Model file for the job. Use its own axes, mm. Face numbers are marked on the shaded views. A direction names the side the tool comes from. Give positions to 0.01 mm unless a question says otherwise; leave off trailing zeros. Write each loop counter-clockwise with the first axis right and the second up, starting at its lowest first coordinate (ties: lowest second). Pieces come first, ordered by that corner, then holes. Notation, with made-up numbers: (71.5, 63) - (94.5, 63) arc R15 cw to (94.5, 90) - close; hole circle Ø4 at (41.5, 53). An arc over 180 degrees is marked (long way). Use a Markdown table: item, result. Add a question column.
```python
from build123d import *

# Parameters (mm, degrees)
ESBO_O1_R                = 1.5
RESSALTO_EXTRUS_O1_DEPTH = 50
ESBO_O2_R                = 2.5
ESBO_O2_W                = 6
ESBO_O2_H                = 10
CORTE_EXTRUS_O2_DEPTH    = 6


with BuildPart() as part:
    # Esboço1 → Ressalto-extrusão1 (new body)
    with BuildSketch(Plane.XY):
        with BuildLine():
            Line((0, 0), (-20, 0))
            ThreePointArc((-20, 0), (-22.324602514, 3.419903881), (-18.2892713, 4.32302148))
            ThreePointArc((-18.2892713, 4.32302148), (-17.800459182, 3.688284557), (-17.537523452, 2.9315197))
            ThreePointArc((-17.537523452, 2.9315197), (-16.656985327, 1.403588896), (-15, 0.8))
            Line((-15, 0.8), (0, 0.8))
            Line((0, 0.8), (0, 0))
        make_face()
        with Locations((-20, 2.5)):
            Circle(ESBO_O1_R, mode=Mode.SUBTRACT)
    extrude(amount=RESSALTO_EXTRUS_O1_DEPTH)

    # Esboço2 → Corte-extrusão2 (cut, through all)
    with BuildSketch(Plane.XZ):
        with Locations((-8, 43)):
            Circle(ESBO_O2_R)
        with Locations((-8, 7)):
            Circle(ESBO_O2_R)
        with Locations((-19.5, 5)):
            Rectangle(ESBO_O2_W, ESBO_O2_H)
        with Locations((-19.5, 25)):
            Rectangle(ESBO_O2_W, ESBO_O2_H)
        with Locations((-19.5, 45)):
            Rectangle(ESBO_O2_W, ESBO_O2_H)
    extrude(amount=-CORTE_EXTRUS_O2_DEPTH, mode=Mode.SUBTRACT)


solid = part.part
```
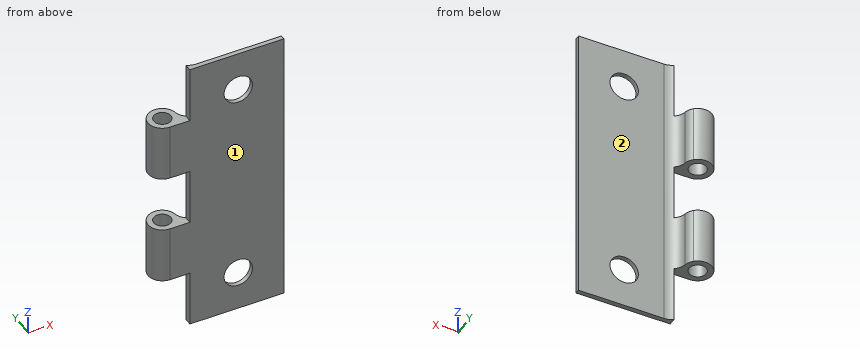
(1) Flat gauge pins, fed straight in: pin 1 (1.4 mm diameter, centred on y = 0.5, z = 25.5, fed in from -X); pin 2 (2.5 mm diameter, centred on x = -18.5, y = 3.5, fed in from -Z); pin 3 (2.5 mm diameter, centred on x = -20, y = 2.5, fed in from +Z); pin 4 (12 mm diameter, centred on x = -10, z = 23, fed in from +Y). Where does each tip first touch, or does it go through?
(2) Probe probe 1 along Z at (x, y) = (-8, 0.25); probe 2 along Z at (x, y) = (-7.25, 0.7); probe 3 along Z at (x, y) = (-21, 0.45). List the from-to ranges inside material, lowest first. Write a range as [from, to].
(3) Band-saw the part on D-D (z = 47). Write the cut outline in (x, y).
(4) Band-saw the part on B-B (x = -8). Write the cut outline in (y, z), then the cut area to 3 significant figures.
(5) Which spindle directions (+Z, -Z, +X, -X, +Y, -Y) get a long thin tool onto all of the face, cutting with end or side? Do the marked faces 1 and 2. Say none if no direction does.
(6) Band-saw the part on C-C (x = -17). Write the cut outline in (y, z), then the cut area to 3 significant figures.
(7) Band-saw the part on A-A (z = 5). Write the cut outline in (x, y).
Model answer:
| question | item | result |
|---|---|---|
| 1 | pin 1 | stops at x = -16.5 |
| 1 | pin 2 | stops at z = 10 |
| 1 | pin 3 | passes through |
| 1 | pin 4 | stops at y = 1 |
| 2 | probe 1 | z = [0, 4.5], [9.5, 40.5], [45.5, 50] |
| 2 | probe 2 | z = [0, 4.62], [9.38, 40.62], [45.38, 50] |
| 2 | probe 3 | z = [10, 20], [30, 40] |
| 3 | outline | (-16.5, 0) - (0, 0) - (0, 0.8) - (-15, 0.8) arc R2.58 cw to (-16.5, 1.28) - close |
| 4 | outline | (0, 0) - (0.8, 0) - (0.8, 4.5) - (0, 4.5) - close; (0, 9.5) - (0.8, 9.5) - (0.8, 40.5) - (0, 40.5) - close; (0, 45.5) - (0.8, 45.5) - (0.8, 50) - (0, 50) - close |
| 4 | area | 32.0 mm^2 |
| 5 | face 1 | +Z, -Z, +X, -X, -Y |
| 5 | face 2 | +Z, -Z, +X, +Y |
| 6 | outline | (0, 10) - (1.75, 10) - (1.75, 20) - (0, 20) - close; (0, 30) - (1.75, 30) - (1.75, 40) - (0, 40) - close |
| 6 | area | 35.0 mm^2 |
| 7 | outline | (-16.5, 0) - (-9.5, 0) - (-9.5, 0.8) - (-15, 0.8) arc R2.58 cw to (-16.5, 1.28) - close; (-6.5, 0) - (0, 0) - (0, 0.8) - (-6.5, 0.8) - close |
